Source: CAD feature listing. Evaluate the final solid. Frame: model axes, mm. Face numbers are marked on the shaded views. Give positions to 0.01 mm unless a question says otherwise; leave off trailing zeros. Order: outer loops, then holes, each group sorted by start corner. A loop starts at its lowest first (then second) coordinate and runs counter-clockwise, first axis right, second up.
1) Material intervals for line 1 (Y direction, x = 6.5, z = 0); line 2 (X direction, y = -3.6, z = 0); line 3 (Z direction, x = 10.5, y = 0.5), sorted ascending.
2) Section A-A, the plane x = 11.5. Return loops of the section in (y, z), plus the area to 3 significant figures.
3) First-contact query: P1, Ø1, axis at x = 1.5, z = -1.5, coming from the -Y side; P2, Ø1, axis at y = 3.5, z = 1.5, coming from the -X side; P3, Ø1.5, axis at x = 10.5, z = -2.5, coming from the -Y side. Flat tips, straight axial feed; report the tip coordinate or a pass-through.
4) Draft query along X for the marked faces 1, 2 and 3. Return one class per face: released by +X, released by -X, zero draft, split by the parting line, or undercut.
5) Section B-B, the plane z = 0. Give the number of separate pieces and of enclosed holes in the cut face, plus the area to 3 significant figures.
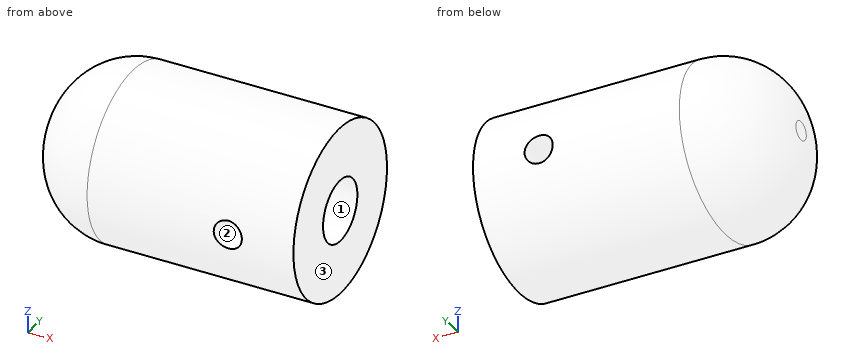
Autodesk Inventor part; units mm, degrees
ref_plane "YZ Plane" through (0, 0, 0) normal (1, 0, 0) x (0, 1, 0)
ref_plane "XZ Plane" through (0, 0, 0) normal (0, 1, 0) x (-1, 0, 0)
ref_plane "XY Plane" through (0, 0, 0) normal (0, 0, 1) x (1, 0, 0)
sketch "スケッチ1" plane through (0, 0, 0) normal (1, 0, 0) x (0, 1, 0)
  circle A0 centre (0, 0) radius 4.5
  dimension "d0" = 9
extrude "押し出し1" add sketch "スケッチ1" along normal blind 15
sketch "スケッチ2" plane through (15, 0, 0) normal (1, 0, 0) x (0, 0, -1)
  circle A0 centre (0, 0) radius 4.5
  circle A1 centre (0, 0) radius 1.65
  dimension "d3" = 3.3
extrude "押し出し2" cut sketch "スケッチ2" against normal blind 13 contours A1
fillet "フィレット1" radius 4 1 edges at (0, -4.5, 0)
sketch "スケッチ3" plane through (0, 0, 0) normal (0, 1, 0) x (-1, 0, 0)
  circle A0 centre (-11.5, 0) radius 0.75
  line L0 (-15, 4.5) -> (-15, -4.5)
  point P0 (0, 0)
  point P1 (-5, -5)
  point P2 (-5, 5)
  dimension "d7" = 1.5
  dimension "d8" = 3.5
  dimension "d9" = 0
extrude "押し出し3" cut sketch "スケッチ3" along normal mid plane 13
properties part number "motor-stick-cap"
From the geometry:
1. line 1: y = -4.5 to -1.65, 1.65 to 4.5
1. line 2: x = 1.47 to 10.75, 12.25 to 15
1. line 3: z = -4.47 to -1.57, 1.57 to 4.47
2. outline: (-4.44, -0.75) arc R4.5 ccw to (4.44, -0.75) - (1.47, -0.75) arc R1.65 cw to (-1.47, -0.75) - close; (-4.44, 0.75) - (-1.47, 0.75) arc R1.65 cw to (1.47, 0.75) - (4.44, 0.75) arc R4.5 ccw to start
2. area: 46.4 mm2
3. P1: stops at y = -3.72
3. P2: stops at x = 1.15
3. P3: stops at y = -4.15
4. face 1: zero draft
4. face 2: undercut
4. face 3: released by +X
5. separate pieces: 3
5. enclosed holes: 0
5. area: 76.7 mm2
